Geometry check sheet. Reference: the model listing, model coordinates, mm. Give positions to 0.01 mm unless a question says otherwise; leave off trailing zeros. Order: outer loops, then holes, each group sorted by start corner. A loop starts at its lowest first (then second) coordinate and runs counter-clockwise, first axis right, second up.
from build123d import *

# Parameters (mm, degrees)
SKETCH1_W               = 111
SKETCH1_H               = 30
BOSS_EXTRUDE1_DEPTH     = 1.5
SKETCH2_W               = 30
SKETCH2_H               = 3
BOSS_EXTRUDE2_DEPTH     = 1.5
CUT_EXTRUDE2_DEPTH      = 59.365229375
CUT_EXTRUDE2_DEPTH_BACK = 59.365229375
CUT_EXTRUDE3_DEPTH      = 59.365229375
CUT_EXTRUDE3_DEPTH_BACK = 59.365229375
SKETCH6_W               = 2
SKETCH6_H               = 4
CUT_EXTRUDE4_DEPTH      = 59.423026282
CUT_EXTRUDE4_DEPTH_BACK = 59.423026282
SKETCH7_W               = 30
SKETCH7_H               = 3
CUT_EXTRUDE5_DEPTH      = 59.365229375
CUT_EXTRUDE5_DEPTH_BACK = 59.365229375
SKETCH8_W               = 85
SKETCH8_H               = 3
CUT_EXTRUDE7_DEPTH      = 59.365229375
CUT_EXTRUDE7_DEPTH_BACK = 59.365229375
SKETCH10_W              = 73
SKETCH10_H              = 8
FILLET1_R               = 3
CUT_EXTRUDE6_DEPTH      = 59.365229375
CUT_EXTRUDE6_DEPTH_BACK = 59.365229375


with BuildPart() as part:
    # Sketch1 → Boss-Extrude1 (new, symmetric)
    with BuildSketch(Plane(origin=(0, 0, 0), x_dir=(1, 0, 0), z_dir=(0, 1, 0))):
        Rectangle(SKETCH1_W, SKETCH1_H)
    extrude(amount=BOSS_EXTRUDE1_DEPTH, both=True)

    # Sketch2 → Boss-Extrude2 (add, symmetric)
    with BuildSketch(Plane(origin=(0, 0, 0), x_dir=(1, 0, 0), z_dir=(0, 1, 0))):
        with Locations((-27.75, -16.5)):
            Rectangle(SKETCH2_W, SKETCH2_H)
        with Locations((27.75, -16.5)):
            Rectangle(SKETCH2_W, SKETCH2_H)
    extrude(amount=BOSS_EXTRUDE2_DEPTH, both=True)

    # Sketch5 → Cut-Extrude2 (cut, two sides: drawn at the far end of the back side and taken through both)
    with BuildSketch(Plane(origin=(0, 0, 0), x_dir=(1, 0, 0), z_dir=(0, 1, 0)).offset(-CUT_EXTRUDE2_DEPTH_BACK)):
        with BuildLine():
            Line((-29.25, -18), (-26.25, -18))
            Line((-26.25, -18), (-26.25, -14))
            Line((-26.25, -14), (-24.9, -14))
            Line((-24.9, -14), (-24.9, -11.73))
            Line((-24.9, -11.73), (-26.25, -11.73))
            Line((-26.25, -11.73), (-26.25, -9))
            ThreePointArc((-26.25, -9), (-26.542893219, -8.292893219), (-27.25, -8))
            Line((-27.25, -8), (-28.25, -8))
            ThreePointArc((-28.25, -8), (-28.957106781, -8.292893219), (-29.25, -9))
            Line((-29.25, -9), (-29.25, -11.73))
            Line((-29.25, -11.73), (-30.596948556, -11.73))
            Line((-30.596948556, -11.73), (-30.596948556, -14))
            Line((-30.596948556, -14), (-29.25, -14))
            Line((-29.25, -14), (-29.25, -18))
        make_face()
        with BuildLine():
            Line((26.25, -14), (24.9, -14))
            Line((24.9, -14), (24.9, -11.73))
            Line((24.9, -11.73), (26.25, -11.73))
            Line((26.25, -11.73), (26.25, -9))
            ThreePointArc((26.25, -9), (26.542893219, -8.292893219), (27.25, -8))
            Line((27.25, -8), (28.25, -8))
            ThreePointArc((28.25, -8), (28.957106781, -8.292893219), (29.25, -9))
            Line((29.25, -9), (29.25, -11.73))
            Line((29.25, -11.73), (30.596948556, -11.73))
            Line((30.596948556, -11.73), (30.596948556, -14))
            Line((30.596948556, -14), (29.25, -14))
            Line((29.25, -14), (29.25, -18))
            Line((29.25, -18), (26.25, -18))
            Line((26.25, -18), (26.25, -14))
        make_face()
    extrude(amount=CUT_EXTRUDE2_DEPTH + CUT_EXTRUDE2_DEPTH_BACK, mode=Mode.SUBTRACT)

    # Sketch6 → Cut-Extrude3 (cut, two sides: drawn at the far end of the back side and taken through both)
    with BuildSketch(Plane(origin=(0, 0, 0), x_dir=(1, 0, 0), z_dir=(0, 1, 0)).offset(-CUT_EXTRUDE3_DEPTH_BACK)):
        with Locations((54.5, -10)):
            Rectangle(SKETCH6_W, SKETCH6_H)
        with Locations((54.5, 3)):
            Rectangle(SKETCH6_W, SKETCH6_H)
    extrude(amount=CUT_EXTRUDE3_DEPTH + CUT_EXTRUDE3_DEPTH_BACK, mode=Mode.SUBTRACT)

    # Sketch7 → Cut-Extrude4 (cut, two sides: drawn at the far end of the back side and taken through both)
    with BuildSketch(Plane(origin=(0, 1.5, 0), x_dir=(1, 0, 0), z_dir=(0, 1, 0)).offset(-CUT_EXTRUDE4_DEPTH_BACK)):
        with Locations((-23.5, -3.5)):
            Rectangle(SKETCH7_W, SKETCH7_H)
        with Locations((23.5, -3.5)):
            Rectangle(SKETCH7_W, SKETCH7_H)
    extrude(amount=CUT_EXTRUDE4_DEPTH + CUT_EXTRUDE4_DEPTH_BACK, mode=Mode.SUBTRACT)

    # Sketch8 → Cut-Extrude5 (cut, two sides: drawn at the far end of the back side and taken through both)
    with BuildSketch(Plane(origin=(0, 0, 0), x_dir=(1, 0, 0), z_dir=(0, 1, 0)).offset(-CUT_EXTRUDE5_DEPTH_BACK)):
        with Locations((0, 13.5)):
            Rectangle(SKETCH8_W, SKETCH8_H)
    extrude(amount=CUT_EXTRUDE5_DEPTH + CUT_EXTRUDE5_DEPTH_BACK, mode=Mode.SUBTRACT)

    # Sketch10 → Cut-Extrude7 (cut, two sides: drawn at the far end of the back side and taken through both)
    with BuildSketch(Plane(origin=(0, 0, 0), x_dir=(1, 0, 0), z_dir=(0, 1, 0)).offset(-CUT_EXTRUDE7_DEPTH_BACK)):
        with Locations((0, 8)):
            Rectangle(SKETCH10_W, SKETCH10_H)
    extrude(amount=CUT_EXTRUDE7_DEPTH + CUT_EXTRUDE7_DEPTH_BACK, mode=Mode.SUBTRACT)

    # Fillet1
    fillet1_edges = [part.edges().sort_by_distance(p)[0] for p in [
        (-36.5, 0, -4),
        (-36.5, 0, -12),
        (36.5, 0, -12),
        (36.5, 0, -4),
    ]]
    fillet(fillet1_edges, radius=FILLET1_R)

    # Sketch9 → Cut-Extrude6 (cut, two sides: drawn at the far end of the back side and taken through both)
    with BuildSketch(Plane(origin=(0, 0, 0), x_dir=(1, 0, 0), z_dir=(0, 1, 0)).offset(-CUT_EXTRUDE6_DEPTH_BACK)):
        with BuildLine():
            Line((-50.5, 15), (-47.5, 15))
            Line((-47.5, 15), (-47.5, 11))
            Line((-47.5, 11), (-46.15, 11))
            Line((-46.15, 11), (-46.15, 8.73))
            Line((-46.15, 8.73), (-47.5, 8.73))
            Line((-47.5, 8.73), (-47.5, 4))
            ThreePointArc((-47.5, 4), (-47.792893219, 3.292893219), (-48.5, 3))
            Line((-48.5, 3), (-49.5, 3))
            ThreePointArc((-49.5, 3), (-50.207106781, 3.292893219), (-50.5, 4))
            Line((-50.5, 4), (-50.5, 8.73))
            Line((-50.5, 8.73), (-51.85, 8.73))
            Line((-51.85, 8.73), (-51.85, 11))
            Line((-51.85, 11), (-50.5, 11))
            Line((-50.5, 11), (-50.5, 15))
        make_face()
        with BuildLine():
            Line((47.5, 8.73), (47.5, 4))
            ThreePointArc((47.5, 4), (47.792893219, 3.292893219), (48.5, 3))
            Line((48.5, 3), (49.5, 3))
            ThreePointArc((49.5, 3), (50.207106781, 3.292893219), (50.5, 4))
            Line((50.5, 4), (50.5, 8.73))
            Line((50.5, 8.73), (51.85, 8.73))
            Line((51.85, 8.73), (51.85, 11))
            Line((51.85, 11), (50.5, 11))
            Line((50.5, 11), (50.5, 15))
            Line((50.5, 15), (47.5, 15))
            Line((47.5, 15), (47.5, 11))
            Line((47.5, 11), (46.15, 11))
            Line((46.15, 11), (46.15, 8.73))
            Line((46.15, 8.73), (47.5, 8.73))
        make_face()
    extrude(amount=CUT_EXTRUDE6_DEPTH + CUT_EXTRUDE6_DEPTH_BACK, mode=Mode.SUBTRACT)


solid = part.part
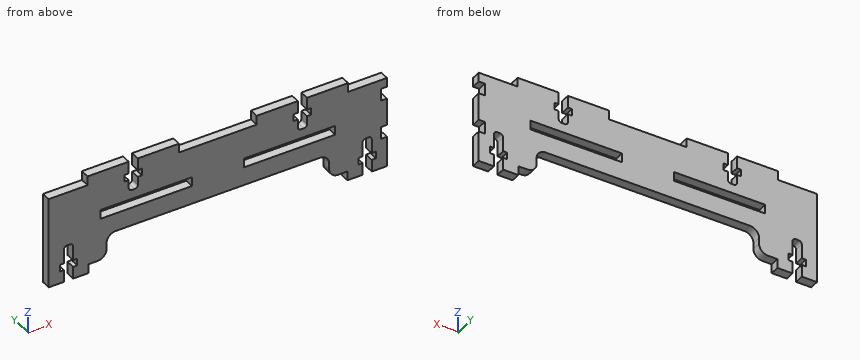
Item 1: Sectioned sample at A-A (z = 16.5). Enter the section's corners in (x, y).
Reported:
outline: (-42.75, -1.5) - (-29.25, -1.5) - (-29.25, 1.5) - (-42.75, 1.5) - close; (-26.25, -1.5) - (-12.75, -1.5) - (-12.75, 1.5) - (-26.25, 1.5) - close; (12.75, -1.5) - (26.25, -1.5) - (26.25, 1.5) - (12.75, 1.5) - close; (29.25, -1.5) - (42.75, -1.5) - (42.75, 1.5) - (29.25, 1.5) - close
Item 2: Sectioned sample at D-D (y = 0.15). Give the number of separate pieces and of enclosed holes in the cut face, and give its area (3 significant figures).
Reported:
separate pieces: 1
enclosed holes: 2
area: 2,320 mm2
Item 3: Sectioned sample at B-B (z = 3.5). Enter the section's corners in (x, y), and give its area (3 significant figures).
Reported:
outline: (-55.5, -1.5) - (-38.5, -1.5) - (-38.5, 1.5) - (-55.5, 1.5) - close; (-8.5, -1.5) - (8.5, -1.5) - (8.5, 1.5) - (-8.5, 1.5) - close; (38.5, -1.5) - (55.5, -1.5) - (55.5, 1.5) - (38.5, 1.5) - close
area: 153 mm2
Item 4: Gauge pin test, flat ends, axial feed: pin 1 (0.5 mm diameter, centred on x = 28, y = 0, fed in from +Z); pin 2 (1.5 mm diameter, centred on x = 41.5, y = 0, fed in from -Z); pin 3 (0.9 mm diameter, centred on y = 0, z = 16, fed in from -X). Record the tip position at first contact, or that the pin passes through.
Reported:
pin 1: stops at z = 8
pin 2: stops at z = -12
pin 3: stops at x = -42.75
Item 5: Scan lines: L1, parallel to X at y = 1, z = 3; L2, parallel to X at y = 0.75, z = 16; L3, parallel to Z at x = -30, y = -1.2. Record each from-to range of solid material in increasing order.
Reported:
L1: x = -55.5 to -38.5, -8.5 to 8.5, 38.5 to 55.5
L2: x = -42.75 to -29.25, -26.25 to -12.75, 12.75 to 26.25, 29.25 to 42.75
L3: z = -4 to 2, 5 to 11.73, 14 to 18
Item 6: Sectioned sample at C-C (x = -18). Enter the section's corners in (y, z), and give its area (3 significant figures).
Reported:
outline: (-1.5, -4) - (1.5, -4) - (1.5, 2) - (-1.5, 2) - close; (-1.5, 5) - (1.5, 5) - (1.5, 18) - (-1.5, 18) - close
area: 57.0 mm2
